Build history of the part. All positions in model axes, mm. Face numbers are marked on the shaded views. Give positions to 0.01 mm unless a question says otherwise; leave off trailing zeros. Order: outer loops, then holes, each group sorted by start corner. A loop starts at its lowest first (then second) coordinate and runs counter-clockwise, first axis right, second up. Notation, with made-up numbers: (-32, -34) - (-23, -34) arc R27 ccw to (-23, -8) - close; hole circle Ø10 at (9, -16.5). An arc over 180 degrees is marked (long way). Answer in a Markdown table with one row per item.
```python
from build123d import *

# Parameters (mm, degrees)
SKETCH3_R           = 20
SKETCH3_W           = 100
SKETCH3_H           = 6
BOSS_EXTRUDE3_DEPTH = 10
SKETCH5_R           = 30
BOSS_EXTRUDE4_DEPTH = 5


with BuildPart() as part:
    # Sketch3 → Boss-Extrude3 (new body)
    with BuildSketch(Plane.XY):
        with Locations((-20.605993479, -1.21989897)):
            Circle(SKETCH3_R)
        with Locations((-0.535964706, -0.268513697)):
            Rectangle(SKETCH3_W, SKETCH3_H)
    extrude(amount=-BOSS_EXTRUDE3_DEPTH)

    # Sketch5 → Boss-Extrude4 (add)
    with BuildSketch(Plane.XY):
        with BuildLine():
            Line((26.021713598, 50.989840857), (-0.622690446, 21.155703813))
            ThreePointArc((-0.622690446, 21.155703813), (6.775561362, 11.037770242), (9.394006521, -1.21989897))
            ThreePointArc((9.394006521, -1.21989897), (6.945592722, -13.090454889), (0, -23.023408613))
            Line((0, -23.023408613), (27.474657971, -52.094754804))
            ThreePointArc((27.474657971, -52.094754804), (49.464035294, -0.232284347), (26.021713598, 50.989840857))
        make_face()
        with Locations((-20.605993479, -1.21989897)):
            Circle(SKETCH5_R)
    extrude(amount=-BOSS_EXTRUDE4_DEPTH)


solid = part.part
```
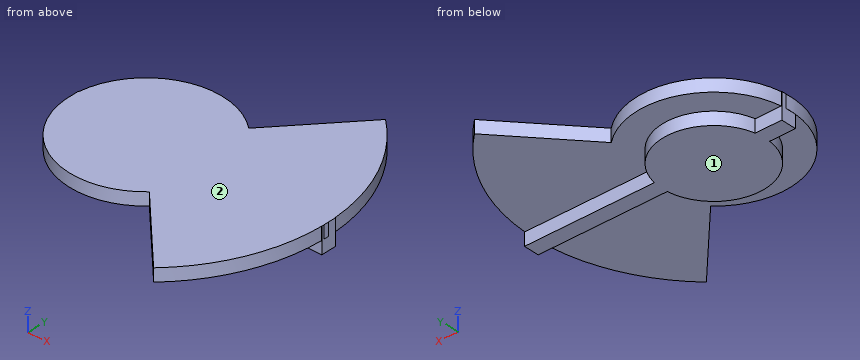
1. Cut at D-D on y = 7. Write the cut outline in (x, z), and give its area (3 significant figures).
Check result:
| item | result |
|---|---|
| outline | (-49.46, -5) - (-38.84, -5) - (-38.84, -10) - (-2.37, -10) - (-2.37, -5) - (48.99, -5) - (48.99, 0) - (-49.46, 0) - close |
| area | 675 mm² |
2. Drop flat-ended pins along their axis: P1, Ø1.8, axis at y = -1.5, z = -5.5, coming from the -X side; P2, Ø6, axis at y = 40, z = -2.5, coming from the -X side; P3, Ø2, axis at y = 17.5, z = -6.5, coming from the -X side. Give the stop position or say it passes through.
Check result:
| item | result |
|---|---|
| P1 | stops at x = -50.61 |
| P2 | stops at x = 13.53 |
| P3 | stops at x = -29.88 |
3. Cut at A-A on y = 26.5. Write the cut outline in (x, z), and give its area (3 significant figures).
Check result:
| item | result |
|---|---|
| outline | (-32.08, -5) - (-9.13, -5) - (-9.13, 0) - (-32.08, 0) - close; (4.15, -5) - (43.74, -5) - (43.74, 0) - (4.15, 0) - close |
| area | 313 mm² |
4. Probe line 1 (Z direction, x = 17, y = -5); line 2 (Y direction, x = 28, z = -8.5); line 3 (X direction, y = -26, z = -4.5). List the from-to ranges inside material, lowest first.
Check result:
| item | result |
|---|---|
| line 1 | z = -5 to 0 |
| line 2 | y = -3.27 to 2.73 |
| line 3 | x = -37.52 to -3.7, 2.81 to 44.93 |
5. Two-plate mould, pull along Z, no slides. Class the marked faces 1 and 2: +Z half, -Z half, draft (parallel to the pull), parting line (faces both ways), or undercut.
Check result:
| item | result |
|---|---|
| face 1 | -Z half |
| face 2 | +Z half |
6. Cut at B-B on x = -3.5. Write the cut outline in (y, z), and give its area (3 significant figures).
Check result:
| item | result |
|---|---|
| outline | (-25.87, -5) - (-11.58, -5) - (-11.58, -10) - (9.14, -10) - (9.14, -5) - (23.43, -5) - (23.43, 0) - (-25.87, 0) - close |
| area | 350 mm² |
